Check sheet for the modelled part. Datum: model origin and axes. Units: mm. A direction names the side the tool comes from. Give positions to 0.01 mm unless a question says otherwise; leave off trailing zeros. Loops run counter-clockwise (first coordinate to the right, second up) from the corner with the lowest first, then second, coordinate; pieces in that order, holes last. Notation, with made-up numbers: (-38.5, 14) - (-25.5, 14) arc R36 cw to (-25.5, 49) - close; hole circle Ø9 at (19, 32). An arc over 180 degrees is marked (long way). Use CSV: the item, a comma, the result in double quotes.
from build123d import *

# Parameters (mm, degrees)
SZKIC1_W                    = 40
SZKIC1_H                    = 20
SZKIC1_W_2                  = 20
SZKIC1_H_2                  = 40
DODANIE_WYCI_GNI_CIE1_DEPTH = 2
SZKIC2_R                    = 3
WYTNIJ_WYCI_GNI_CIE1_DEPTH  = 2


with BuildPart() as part:
    # Szkic1 → Dodanie-wyciągnięcie1 (new body)
    with BuildSketch(Plane.XY):
        with Locations((-19.435499515, 2.2)):
            Rectangle(SZKIC1_W, SZKIC1_H)
        with Locations((-49.435499515, 2.2)):
            Rectangle(SZKIC1_W_2, SZKIC1_H_2)
    extrude(amount=DODANIE_WYCI_GNI_CIE1_DEPTH)

    # Szkic2 → Wytnij-wyciągnięcie1 (cut)
    with BuildSketch(Plane.XY.offset(2)):
        with Locations((-9.435499515, 2.2)):
            Circle(SZKIC2_R)
        with Locations((-49.435499515, 12.2)):
            Circle(SZKIC2_R)
        with Locations((-49.435499515, -7.8)):
            Circle(SZKIC2_R)
    extrude(amount=-WYTNIJ_WYCI_GNI_CIE1_DEPTH, mode=Mode.SUBTRACT)


solid = part.part
1. Scan lines: line 1 along Y through (x, z) = (-50.5, 1.7); line 2 along Y through (x, z) = (-34.5, 1.85); line 3 along Y through (x, z) = (-48, 1). Record each from-to range of solid material in increasing order.
Completed:
line 1,"y = -17.8 to -10.6, -5 to 9.4, 15 to 22.2"
line 2,"y = -7.8 to 12.2"
line 3,"y = -17.8 to -10.43, -5.17 to 9.57, 14.83 to 22.2"
2. Sectioned sample at C-C, the plane x = -48.5. Record the boundary of the cut face in (y, z), and give its area (3 significant figures).
Completed:
outline,"(-17.8, 0) - (-10.65, 0) - (-10.65, 2) - (-17.8, 2) - close; (-4.95, 0) - (9.35, 0) - (9.35, 2) - (-4.95, 2) - close; (15.05, 0) - (22.2, 0) - (22.2, 2) - (15.05, 2) - close"
area,"57.2 mm²"
3. Sectioned sample at B-B, the plane z = 1.1. Record the boundary of the cut face in (x, y).
Completed:
outline,"(-59.44, -17.8) - (-39.44, -17.8) - (-39.44, -7.8) - (0.56, -7.8) - (0.56, 12.2) - (-39.44, 12.2) - (-39.44, 22.2) - (-59.44, 22.2) - close; hole circle Ø6 at (-49.44, -7.8); hole circle Ø6 at (-49.44, 12.2); hole circle Ø6 at (-9.44, 2.2)"
4. Sectioned sample at D-D, the plane x = -14. Record the boundary of the cut face in (y, z).
Completed:
outline,"(-7.8, 0) - (12.2, 0) - (12.2, 2) - (-7.8, 2) - close"
5. Release check for a two-part mould opening along Y. For faces 1 (the face through (0.565, 2, 1)), 2 (the face through (-20, -7.8, 1)), 3 (the face through (-52.433, 12.332, 1.014)) record: released by +Y, released by -Y, zero draft, split by the parting line, or undercut.
Completed:
face 1,"zero draft"
face 2,"released by -Y"
face 3,"undercut"
6. Go/stop test with flat-tipped pins: pin 1 Ø9.5 at (x, y) = (-9.44, 2.2) entering from -Z; pin 2 Ø1 at (x, z) = (-10.5, 0.5) entering from -Y; pin 3 Ø0.6 at (x, z) = (-27.5, 1) entering from +Y. Record where each tip stops, or that it passes through.
Completed:
pin 1,"stops at z = 0"
pin 2,"stops at y = -7.8"
pin 3,"stops at y = 12.2"
7. Sectioned sample at A-A, the plane y = 2.2. Record the boundary of the cut face in (x, z).
Completed:
outline,"(-59.44, 0) - (-12.44, 0) - (-12.44, 2) - (-59.44, 2) - close; (-6.44, 0) - (0.56, 0) - (0.56, 2) - (-6.44, 2) - close"
8. Set-up check for faces 4 (the face through (-39.435, -13, 1)), 5 (the face through (-39.435, 17, 1)), 6 (the face through (-50, 22.2, 1)): record each of +Z, -Z, +X, -X, +Y, -Y from which the full face is reachable in a straight line by a thin tool's end or side.
Completed:
face 4,"+Z, -Z, +X, -Y"
face 5,"+Z, -Z, +X, +Y"
face 6,"+Z, -Z, +X, -X, +Y"
